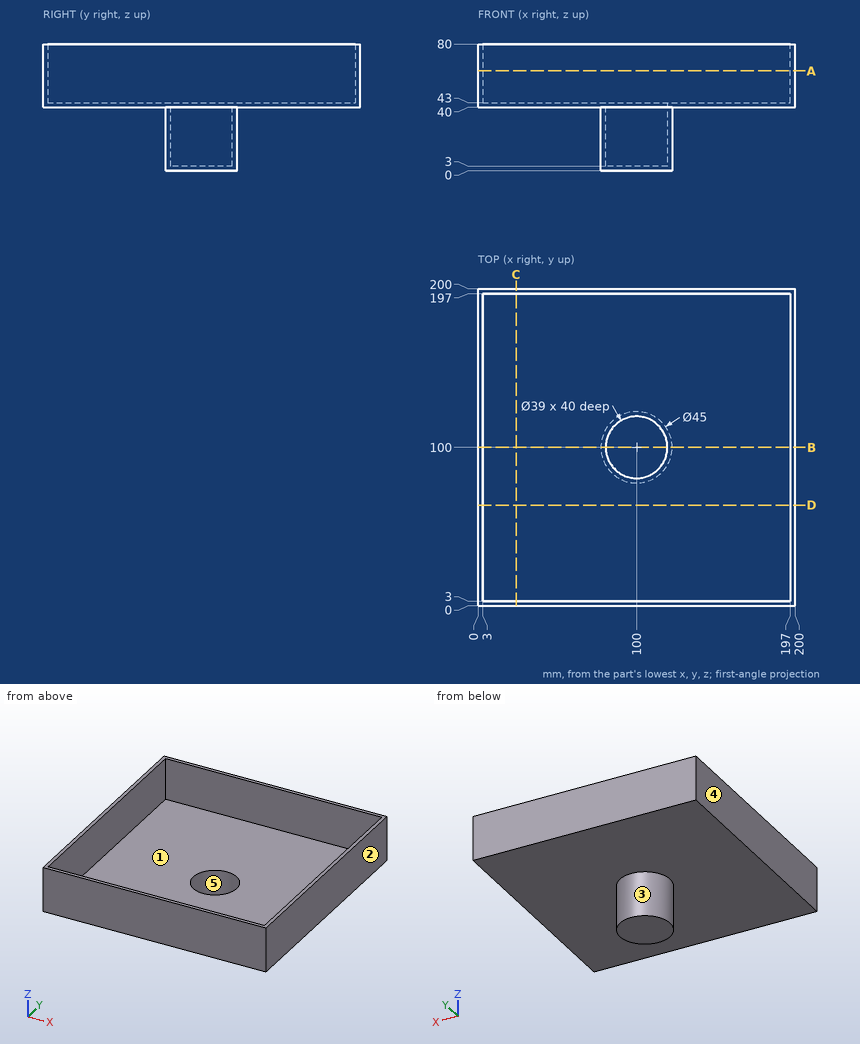
Can you work these out from the drawing? Everything is in mm from the part's minimum corner. A direction names the side the tool comes from. Coordinates: 2 decimals unless noted, no trailing zeros. Loops run counter-clockwise (first coordinate to the right, second up) from the corner with the lowest first, then second, coordinate; pieces in that order, holes last.
1) Which directions (+Z, -Z, +X, -X, +Y, -Y) give clear straight access to the entire face, cutting with the end or side of a thin tool? Please do the marked faces 1 and 2.
Reported:
face 1: +Z
face 2: +Z, -Z, +X, +Y, -Y
2) Imagine slicing it at A-A (z = 63). List the corners of the cut face in (x, y) for me.
Reported:
outline: (0, 0) - (200, 0) - (200, 200) - (0, 200) - close; hole (3, 3) - (197, 3) - (197, 197) - (3, 197) - close
3) Imagine slicing it at B-B (y = 100). List the corners of the cut face in (x, z) for me, and give its area (3 significant figures).
Reported:
outline: (0, 40) - (77.5, 40) - (77.5, 0) - (122.5, 0) - (122.5, 40) - (200, 40) - (200, 80) - (197, 80) - (197, 43) - (119.5, 43) - (119.5, 3) - (80.5, 3) - (80.5, 43) - (3, 43) - (3, 80) - (0, 80) - close
area: 1,060 mm2
4) Thinking about a two-plate mould opening in Y: for the marked faces 3, 4 and 5, which applies, released by +Y, released by -Y, zero draft, split by the parting line, or undercut?
Reported:
face 3: split by the parting line
face 4: zero draft
face 5: undercut
5) Imagine slicing it at C-C (x = 24). List the corners of the cut face in (y, z) for me, and give its area (3 significant figures).
Reported:
outline: (0, 40) - (200, 40) - (200, 80) - (197, 80) - (197, 43) - (3, 43) - (3, 80) - (0, 80) - close
area: 822 mm2
6) Will these pins go through, and if not, where does the flat tip stop? pin 1 Ø8 at (x, z) = (33.5, 32.5) entering from +Y; pin 2 Ø2 at (x, y) = (122.5, 22.5) entering from -Z; pin 3 Ø1.5 at (x, y) = (134.5, 39) entering from +Z; pin 4 Ø11.5 at (x, y) = (98.5, 100.5) entering from +Z.
Reported:
pin 1: passes through
pin 2: stops at z = 40
pin 3: stops at z = 43
pin 4: stops at z = 3
7) Please list where these lines run through material, in increasing order: line 1 along Y through (x, z) = (55.5, 58); line 2 along Y through (x, z) = (100, 24).
Reported:
line 1: y = 0 to 3, 197 to 200
line 2: y = 77.5 to 80.5, 119.5 to 122.5
